Work out the finished part from the listing and answer in its coordinate system (mm). Give positions to 0.01 mm unless a question says otherwise; leave off trailing zeros. Loops run counter-clockwise (first coordinate to the right, second up) from the corner with the lowest first, then second, coordinate; pieces in that order, holes last. Notation, with made-up numbers: (-10, 36) - (10, 36) arc R26 ccw to (10, 75) - close; hole circle Ø7 at (84, 58). An arc over 180 degrees is marked (long way). One line per question, with ' | ' between items.
from build123d import *

# Parameters (mm, degrees)
SKETCH1_R           = 1.25
SKETCH1_W           = 22.686844956
SKETCH1_H           = 12.666164059
BOSS_EXTRUDE1_DEPTH = 1.6


with BuildPart() as part:
    # Sketch1 → Boss-Extrude1 (new body)
    with BuildSketch(Plane(origin=(0, 0, 0), x_dir=(1, 0, 0), z_dir=(0, 1, 0))):
        with BuildLine():
            Line((-18, 21.5), (18, 21.5))
            ThreePointArc((18, 21.5), (20.121320344, 20.621320344), (21, 18.5))
            Line((21, 18.5), (21, -18.5))
            ThreePointArc((21, -18.5), (20.121320344, -20.621320344), (18, -21.5))
            Line((18, -21.5), (-18, -21.5))
            ThreePointArc((-18, -21.5), (-20.121320344, -20.621320344), (-21, -18.5))
            Line((-21, -18.5), (-21, 18.5))
            ThreePointArc((-21, 18.5), (-20.121320344, 20.621320344), (-18, 21.5))
        make_face()
        with Locations((-18.0215, 18.707)):
            Circle(SKETCH1_R, mode=Mode.SUBTRACT)
        with Locations((18.0215, 18.707)):
            Circle(SKETCH1_R, mode=Mode.SUBTRACT)
        with Locations((18.0215, -18.707)):
            Circle(SKETCH1_R, mode=Mode.SUBTRACT)
        with Locations((-18.0215, -18.707)):
            Circle(SKETCH1_R, mode=Mode.SUBTRACT)
        with Locations((0, -27.83308203)):
            Rectangle(SKETCH1_W, SKETCH1_H)
    extrude(amount=BOSS_EXTRUDE1_DEPTH)


solid = part.part
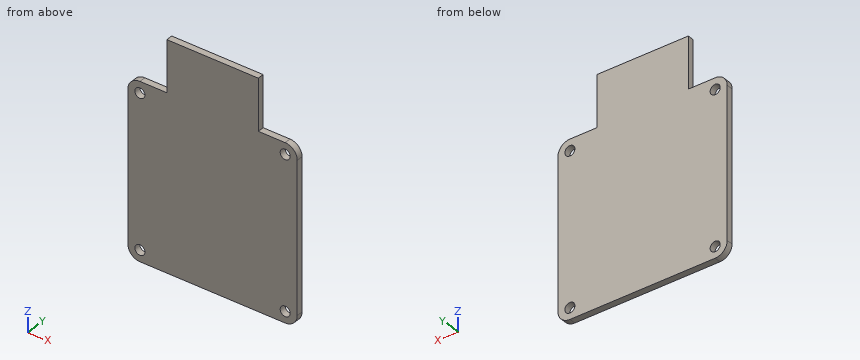
1. Find section A-A on y = 0.35. Write down the section's boundary in (x, z).
Evaluation:
outline: (-21, -18.5) arc R3 ccw to (-18, -21.5) - (18, -21.5) arc R3 ccw to (21, -18.5) - (21, 18.5) arc R3 ccw to (18, 21.5) - (11.34, 21.5) - (11.34, 34.17) - (-11.34, 34.17) - (-11.34, 21.5) - (-18, 21.5) arc R3 ccw to (-21, 18.5) - close; hole circle Ø2.5 at (-18.02, -18.71); hole circle Ø2.5 at (-18.02, 18.71); hole circle Ø2.5 at (18.02, -18.71); hole circle Ø2.5 at (18.02, 18.71)
2. Find section B-B on x = -15.5. Write down the section's boundary in (y, z), then the cut area to 3 significant figures.
Evaluation:
outline: (0, -21.5) - (1.6, -21.5) - (1.6, 21.5) - (0, 21.5) - close | area: 68.8 mm2
3. Consider L1, parallel to Z at x = 14.5, y = 1; L2, parallel to X at y = 0.5, z = 23.5. Determine where each line is inside the solid, lowest interval first.
Evaluation:
L1: -21.5 to 21.5 | L2: -11.34 to 11.34
4. Flat-ended cylindrical pins translate along their axes: pin 1 (2 mm diameter, centred on x = 18.02, z = 18.71, fed in from +Y); pin 2 (0.8 mm diameter, centred on y = 1, z = 30.5, fed in from -X); pin 3 (0.5 mm diameter, centred on x = -13.5, y = 1, fed in from +Z); pin 4 (4 mm diameter, centred on x = -18.02, z = -18.71, fed in from +Y). Find the tip coordinate at first contact, or state that the pin passes through.
Evaluation:
pin 1: through | pin 2: x = -11.34 | pin 3: z = 21.5 | pin 4: y = 1.6
